```python
from build123d import *

# Parameters (mm, degrees)
SKETCH3_W                                        = 226.06
SKETCH3_H                                        = 149.86
EXTRUDE2_DEPTH                                   = 21.844
SKETCH4_W                                        = 226.06
SKETCH4_H                                        = 149.86
SKETCH4_W_2                                      = 22.225
SKETCH4_H_2                                      = 50.8
EXTRUDE4_DEPTH                                   = 0.762
F_1_4_20_TAPPED_HOLE1_D                          = 5.1054
CBORE_FOR_3_8_SOCKET_HEAD_CAP_SCREW1_D           = 10.31748
CBORE_FOR_3_8_SOCKET_HEAD_CAP_SCREW1_CBORE_D     = 38.1
CBORE_FOR_3_8_SOCKET_HEAD_CAP_SCREW1_CBORE_DEPTH = 14.224
SKETCH17_W                                       = 3.175
SKETCH17_H                                       = 133.35
CUT_EXTRUDE1_DEPTH                               = 0.762
CBORE_FOR_1_4_SOCKET_HEAD_CAP_SCREW1_AT_COUNT    = 2
CBORE_FOR_1_4_SOCKET_HEAD_CAP_SCREW1_AT_PITCH    = 63.5
CBORE_FOR_1_4_SOCKET_HEAD_CAP_SCREW1_2_COUNT     = 2
CBORE_FOR_1_4_SOCKET_HEAD_CAP_SCREW1_2_PITCH     = 186.028991356
CBORE_FOR_1_4_SOCKET_HEAD_CAP_SCREW1_3_COUNT     = 2
CBORE_FOR_1_4_SOCKET_HEAD_CAP_SCREW1_3_PITCH     = 166.589197204
F_10_32_TAPPED_HOLE1_D                           = 4.0386
CHAMFER1_SIZE                                    = 12.7


with BuildPart() as part:
    # Sketch3 → Extrude2 (new body)
    with BuildSketch(Plane.XY):
        with Locations((113.03, -74.93)):
            Rectangle(SKETCH3_W, SKETCH3_H)
    extrude(amount=EXTRUDE2_DEPTH)

    # Sketch4 → Extrude4 (cut)
    with BuildSketch(Plane.XY.offset(21.844)):
        with Locations((113.03, -74.93)):
            Rectangle(SKETCH4_W, SKETCH4_H)
        with Locations((30.4927, -116.205)):
            Rectangle(SKETCH4_W_2, SKETCH4_H_2, mode=Mode.SUBTRACT)
        with Locations((30.4927, -33.655)):
            Rectangle(SKETCH4_W_2, SKETCH4_H_2, mode=Mode.SUBTRACT)
        with Locations((195.5673, -116.205)):
            Rectangle(SKETCH4_W_2, SKETCH4_H_2, mode=Mode.SUBTRACT)
        with Locations((195.5673, -33.655)):
            Rectangle(SKETCH4_W_2, SKETCH4_H_2, mode=Mode.SUBTRACT)
    extrude(amount=-EXTRUDE4_DEPTH, mode=Mode.SUBTRACT)

    # 1/4-20 Tapped Hole1 (through all)
    with Locations(Plane(origin=(0, 0, 0), x_dir=(-1, 0, 0), z_dir=(0, 0, -1))):
        with Locations((-195.58, -20.955), (-195.58, -128.905), (-30.48, -43.18), (-30.48, -106.68)):
            Hole(F_1_4_20_TAPPED_HOLE1_D / 2)

    # CBORE for 3/8 Socket Head Cap Screw1 (through all)
    with Locations(Plane.XY.offset(21.082)):
        with Locations((62.23, -125.73), (163.83, -24.13), (62.23, -24.13), (163.83, -125.73)):
            CounterBoreHole(CBORE_FOR_3_8_SOCKET_HEAD_CAP_SCREW1_D / 2, CBORE_FOR_3_8_SOCKET_HEAD_CAP_SCREW1_CBORE_D / 2, CBORE_FOR_3_8_SOCKET_HEAD_CAP_SCREW1_CBORE_DEPTH)

    # Sketch17 → Cut-Extrude1 (cut)
    with BuildSketch(Plane.XY.offset(21.844)):
        with Locations((195.58, -74.93)):
            Rectangle(SKETCH17_W, SKETCH17_H)
        with Locations((30.48, -74.93)):
            Rectangle(SKETCH17_W, SKETCH17_H)
    extrude(amount=-CUT_EXTRUDE1_DEPTH, mode=Mode.SUBTRACT)

    # Sketch19 → CBORE for 1/4 Socket Head Cap Screw1 (revolve, cut)
    with BuildSketch(Plane(origin=(195.58, -106.68, 0), x_dir=(0, 1, 0), z_dir=(1, 0, 0))):
        Polygon((0, 0), (0, 21.844), (3.57124, 21.844), (3.57124, 18.161), (5.55625, 18.161), (5.55625, 0.635), (6.19125, 0), align=None)
    cbore_for_1_4_socket_head_cap_screw1 = revolve(axis=Axis((195.58, -106.68, -6.35), (0, 0, 1)), mode=Mode.SUBTRACT)

    # CBORE for 1/4 Socket Head Cap Screw1 at: CBORE for 1/4 Socket Head Cap Screw1 ×2
    with Locations(*[(0, i * CBORE_FOR_1_4_SOCKET_HEAD_CAP_SCREW1_AT_PITCH, 0) for i in range(1, CBORE_FOR_1_4_SOCKET_HEAD_CAP_SCREW1_AT_COUNT)]):
        add(cbore_for_1_4_socket_head_cap_screw1, mode=Mode.SUBTRACT)

    # CBORE for 1_4 Socket Head Cap Screw1 2: CBORE for 1/4 Socket Head Cap Screw1 ×2
    with Locations(*[Vector(-0.887496077, 0.460815271, 0) * (i * CBORE_FOR_1_4_SOCKET_HEAD_CAP_SCREW1_2_PITCH) for i in range(1, CBORE_FOR_1_4_SOCKET_HEAD_CAP_SCREW1_2_COUNT)]):
        add(cbore_for_1_4_socket_head_cap_screw1, mode=Mode.SUBTRACT)

    # CBORE for 1_4 Socket Head Cap Screw1 3: CBORE for 1/4 Socket Head Cap Screw1 ×2
    with Locations(*[Vector(-0.991060662, -0.133412012, 0) * (i * CBORE_FOR_1_4_SOCKET_HEAD_CAP_SCREW1_3_PITCH) for i in range(1, CBORE_FOR_1_4_SOCKET_HEAD_CAP_SCREW1_3_COUNT)]):
        add(cbore_for_1_4_socket_head_cap_screw1, mode=Mode.SUBTRACT)

    # #10-32 Tapped Hole1 (through all)
    with Locations(Plane(origin=(0, 0, 0), x_dir=(-1, 0, 0), z_dir=(0, 0, -1))):
        with Locations((-100.33, -136.8552), (-125.73, -136.8552), (-113.03, -13.0048)):
            Hole(F_10_32_TAPPED_HOLE1_D / 2)

    # Chamfer1
    chamfer1_edges = [part.edges().sort_by_distance(p)[0] for p in [
        (0, 0, 10.541),
        (226.06, 0, 10.541),
        (226.06, -149.86, 10.541),
        (0, -149.86, 10.541),
    ]]
    chamfer(chamfer1_edges, length=CHAMFER1_SIZE)


solid = part.part
```
CAD build for the part. Positions are in the model's coordinates, mm. A direction names the side the tool comes from. Round coordinates to 2 decimals unless told otherwise and drop trailing zeros. Loops run counter-clockwise (first coordinate to the right, second up) from the corner with the lowest first, then second, coordinate; pieces in that order, holes last. Notation, with made-up numbers: (23.25, -5.75) - (46.25, -5.75) arc R23 cw to (46.25, 4.25) - close; hole circle Ø9 at (69.25, -33). An arc over 180 degrees is marked (long way). Return JSON: item names as keys, results as strings. Group by question number.
Q1. Two-plate mould, pull along Y, no slides. Class faces 4 (the face through (112, 0, 10)), 5 (the face through (112, -149.86, 10)), 6 (the face through (59.46, -121.38, 3.38)), 7 (the face through (111, -74, 0)): +Y half, -Y half, draft (parallel to the pull), parting line (faces both ways), or undercut.
Q2. Band-saw the part on A-A on z = 4. Give the number of separate pieces and of enclosed holes in the cut face, plus the area to 3 significant figures.
Q3. Drill centre lines: line 1 along Y through (x, z) = (195.58, 7.25); line 2 along Y through (x, z) = (195.58, 19.75); line 3 along X through (y, z) = (-39.5, 12.25). Where is each one in solid material? Low to high. Write a range as [from, to].
Q4. Flat gauge pins, fed straight in: pin 1 Ø2.5 at (x, y) = (113.03, -13) entering from +Z; pin 2 Ø5 at (x, y) = (169, -49) entering from -Z; pin 3 Ø2.5 at (x, y) = (195.5, -121.5) entering from +Z; pin 4 Ø0.6 at (y, z) = (-134.5, 21.5) entering from +X. Where does each tip first touch, or does it go through?
Q5. Tool access for faces 1 (the face through (193.554, -130.458, 11.075)), 2 (the face through (168, -28, 6.858)), 3 (the face through (33.861, -133.314, 9.275)): list every direction of +Z, -Z, +X, -X, +Y, -Y with a clear straight run to the whole face (end or side of a thin tool).
Q6. Band-saw the part on B-B on y = -97. Give the cut face in (x, z), plus the area to 3 significant figures.
Q7. Band-saw the part on C-C on x = 79. Give the cut face in (y, z).
Q8. Band-saw the part on D-D on x = 54. Give the cut face in (y, z), plus the area to 3 significant figures.
Solutions:
{
 "1": {"face 4": "+Y half", "face 5": "-Y half", "face 6": "undercut", "face 7": "draft"},
 "2": {"separate pieces": "1", "enclosed holes": "15", "area": "32,700 mm^2"},
 "3": {"line 1": "y = [-149.86, -131.46], [-126.35, -112.24], [-101.12, -48.74], [-37.62, -23.51], [-18.4, 0]", "line 2": "y = [-149.86, -131.46], [-126.35, -110.25], [-103.11, -46.75], [-39.61, -23.51], [-18.4, 0]", "line 3": "x = [0, 50.98], [73.48, 152.58], [175.08, 191.42], [199.74, 226.06]"},
 "4": {"pin 1": "passes through", "pin 2": "stops at z = 0", "pin 3": "stops at z = 21.08", "pin 4": "stops at x = 206.68"},
 "5": {"face 1": "+Z, -Z", "face 2": "+Z", "face 3": "-Z"},
 "6": {"outline": "(0, 0) - (226.06, 0) - (226.06, 21.08) - (206.68, 21.08) - (206.68, 21.84) - (197.17, 21.84) - (197.17, 21.08) - (193.99, 21.08) - (193.99, 21.84) - (184.45, 21.84) - (184.45, 21.08) - (41.61, 21.08) - (41.61, 21.84) - (32.07, 21.84) - (32.07, 21.08) - (28.89, 21.08) - (28.89, 21.84) - (19.38, 21.84) - (19.38, 21.08) - (0, 21.08) - close", "area": "4,790 mm^2"},
 "7": {"outline": "(-149.86, 0) - (0, 0) - (0, 21.08) - (-15.09, 21.08) - (-15.09, 6.86) - (-33.17, 6.86) - (-33.17, 21.08) - (-116.69, 21.08) - (-116.69, 6.86) - (-134.77, 6.86) - (-134.77, 21.08) - (-149.86, 21.08) - close"},
 "8": {"outline": "(-149.86, 0) - (0, 0) - (0, 21.08) - (-6.95, 21.08) - (-6.95, 6.86) - (-41.31, 6.86) - (-41.31, 21.08) - (-108.55, 21.08) - (-108.55, 6.86) - (-142.91, 6.86) - (-142.91, 21.08) - (-149.86, 21.08) - close", "area": "2,180 mm^2"}
}
